Work out the finished part from the listing and answer in its coordinate system (mm). Round coordinates to 2 decimals unless told otherwise and drop trailing zeros. Loops run counter-clockwise (first coordinate to the right, second up) from the corner with the lowest first, then second, coordinate; pieces in that order, holes last.
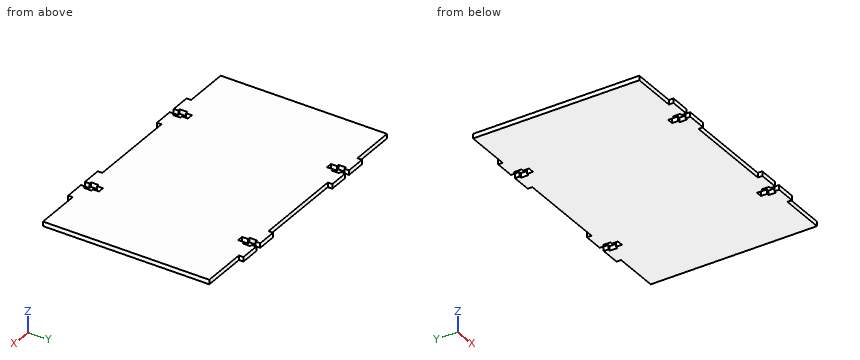
```python
from build123d import *

# Parameters (mm, degrees)
EXTRUDE_1_DEPTH = 3


with BuildPart() as part:
    # 草图1 → 凸台-拉伸1 (new body)
    with BuildSketch(Plane.XY):
        Polygon((90, -55), (90, 0), (60, 0), (48.5, 0), (48.5, -5), (47, -5), (47, -9), (43, -9), (43, -5), (41.5, -5), (41.5, 0), (30, 0), (0, 0), (0, -55), align=None)
        Polygon((120, 0), (90, 0), (90, -55), (180, -55), (180, 0), (150, 0), (138.5, 0), (138.5, -5), (137, -5), (137, -9), (133, -9), (133, -5), (131.5, -5), (131.5, 0), align=None)
        Polygon((180, -55), (90, -55), (90, -110), (120, -110), (131.5, -110), (131.5, -105), (133, -105), (133, -101), (137, -101), (137, -105), (138.5, -105), (138.5, -110), (150, -110), (180, -110), align=None)
        Polygon((90, -110), (90, -55), (0, -55), (0, -110), (30, -110), (41.5, -110), (41.5, -105), (43, -105), (43, -101), (47, -101), (47, -105), (48.5, -105), (48.5, -110), (60, -110), align=None)
        Polygon((120, 3), (120, 0), (131.5, 0), (133, 0), (133, 3), align=None)
        Polygon((138.5, 0), (150, 0), (150, 3), (137, 3), (137, 0), align=None)
        Polygon((30, 3), (30, 0), (41.5, 0), (43, 0), (43, 3), align=None)
        Polygon((48.5, 0), (60, 0), (60, 3), (47, 3), (47, 0), align=None)
        Polygon((60, -113), (60, -110), (48.5, -110), (47, -110), (47, -113), align=None)
        Polygon((41.5, -110), (30, -110), (30, -113), (43, -113), (43, -110), align=None)
        Polygon((150, -113), (150, -110), (138.5, -110), (137, -110), (137, -113), align=None)
        Polygon((131.5, -110), (120, -110), (120, -113), (133, -113), (133, -110), align=None)
    extrude(amount=EXTRUDE_1_DEPTH)


solid = part.part
```
1. Consider probe 1 along Y at (x, z) = (137.5, 2); probe 2 along X at (y, z) = (-106, 1.45); probe 3 along Y at (x, z) = (169.5, 1.6). Determine where each line is inside the solid, lowest interval first.
Answer key:
probe 1: y = -113 to -110, -105 to -5, 0 to 3
probe 2: x = 0 to 41.5, 48.5 to 131.5, 138.5 to 180
probe 3: y = -110 to 0
2. Given pin 1 (1.5 mm diameter, centred on x = 104, z = 1.5, fed in from -Y); pin 2 (0.9 mm diameter, centred on y = 1.5, z = 1.5, fed in from +X), each flat-ended and moving along its own axis, determine where each tip first touches the part or whether it passes through.
Answer key:
pin 1: stops at y = -110
pin 2: stops at x = 150
3. Find section A-A (x = 70). Write down the section's boundary in (y, z), then the cut area to 3 significant figures.
Answer key:
outline: (-110, 0) - (0, 0) - (0, 3) - (-110, 3) - close
area: 330 mm2
